from build123d import *

# Parameters (mm, degrees)
SKETCH1_W           = 1090
SKETCH1_H           = 20
BOSS_EXTRUDE1_DEPTH = 1
BOSS_EXTRUDE4_DEPTH = 1090
SKETCH5_W           = 1090
SKETCH5_H           = 1
BOSS_EXTRUDE5_DEPTH = 582
BOSS_EXTRUDE6_DEPTH = 1090
SKETCH7_W           = 1089
SKETCH7_H           = 1
BOSS_EXTRUDE7_DEPTH = 106


with BuildPart() as part:
    # Sketch1 → Boss-Extrude1 (new body)
    with BuildSketch(Plane(origin=(0, 0, 0), x_dir=(1, 0, 0), z_dir=(0, 1, 0))):
        Rectangle(SKETCH1_W, SKETCH1_H)
    extrude(amount=BOSS_EXTRUDE1_DEPTH)

    # Sketch4 → Boss-Extrude4 (add)
    with BuildSketch(Plane.ZY.offset(545)):
        with BuildLine():
            Line((-10, 1), (-10.77384021, 0.366619127))
            ThreePointArc((-10.77384021, 0.366619127), (-10.428146661, 0.096290735), (-10, 0))
            Line((-10, 0), (-10, 1))
        make_face()
    extrude(amount=-BOSS_EXTRUDE4_DEPTH)

    # Sketch5 → Boss-Extrude5 (add)
    with BuildSketch(Plane(origin=(0, 5.500184543, -4.501848885), x_dir=(1, 0, 0), z_dir=(0, 0.7738402097265024, -0.6333808726275547))):
        with Locations((0, 7.605021225)):
            Rectangle(SKETCH5_W, SKETCH5_H)
    extrude(amount=BOSS_EXTRUDE5_DEPTH)

    # Sketch6 → Boss-Extrude6 (add)
    with BuildSketch(Plane(origin=(545, 0, 0), x_dir=(0, 0, -1), z_dir=(1, 0, 0))):
        with BuildLine():
            Line((378.627667869, 451.375002061), (379.627667869, 451.375002061))
            ThreePointArc((379.627667869, 451.375002061), (379.569432227, 451.038728519), (379.401508079, 450.741621188))
            Line((379.401508079, 450.741621188), (378.627667869, 451.375002061))
        make_face()
    extrude(amount=-BOSS_EXTRUDE6_DEPTH)

    # Sketch7 → Boss-Extrude7 (add)
    with BuildSketch(Plane(origin=(0, 451.375002061, 0), x_dir=(1, 0, 0), z_dir=(0, 1, 0))):
        with Locations((0.5, 379.127667869)):
            Rectangle(SKETCH7_W, SKETCH7_H)
    extrude(amount=BOSS_EXTRUDE7_DEPTH)


solid = part.part
Input: part model. Units: mm. Frame: model coordinates. A direction names the side the tool comes from. Round coordinates to 2 decimals unless told otherwise and drop trailing zeros. Loops run counter-clockwise (first coordinate to the right, second up) from the corner with the lowest first, then second, coordinate; pieces in that order, holes last. Notation, with made-up numbers: (28, 72.25) -> (77, 72.25) arc R30 ccw to (77, 98.25) -> close; hole circle Ø8 at (3.25, 26.25). An arc over 180 degrees is marked (long way). Answer as a JSON object with one key per item and string values. Group by question number.
1) Pin query (flat end, axial travel): pin 1 (12 mm diameter, centred on x = -92, z = -243, fed in from +Y); pin 2 (0.5 mm diameter, centred on x = -544.5, z = -379, fed in from +Y) (3 decimals); pin 3 (12 mm diameter, centred on x = 100.5, z = -102, fed in from -Y). Return the tip coordinate at first contact, or that it passes through.
2) Reachability of faces 1 (the flat face through (-8, 0, 0)), 2 (the flat face through (-8, 1, 0)) from +Z, -Z, +X, -X, +Y, -Y: full face, straight path, thin tool, end or side. Return the list, or none.
3) Ray query, L1, parallel to Z at x = 193, y = 515.5; L2, parallel to Y at x = 340.5, z = -83; L3, parallel to Y at x = 304, z = -221. Return the intervals inside material, ascending.
4) Section query A-A on x = -269.5. Output: boundary loops of the cut face in (y, z) (1 decimal).
5) Section query C-C on z = -115.5. Output: boundary loops of the cut face in (x, y), plus the area to 3 significant figures.
6) Section query B-B on y = 258.5. Output: boundary loops of the cut face in (x, z), plus the area to 3 significant figures.
Reply:
{
 "1": {"pin 1": "stops at y = 293", "pin 2": "stops at y = 451.375", "pin 3": "stops at y = 104.49"},
 "2": {"face 1": "+Z, -Z, +X, -X, -Y", "face 2": "+Z, +X, -X, +Y"},
 "3": {"L1": "z = -379.63 to -378.63", "L2": "y = 88.61 to 90.19", "L3": "y = 257.21 to 258.79"},
 "4": {"outline": "(0, -10) arc R1 ccw to (0.4, -10.8) -> (450.7, -379.4) arc R1 ccw to (451.4, -379.6) -> (557.4, -379.6) -> (557.4, -378.6) -> (451.4, -378.6) -> (1, -10) -> (1, 10) -> (0, 10) -> close"},
 "5": {"outline": "(-545, 128.32) -> (545, 128.32) -> (545, 129.9) -> (-545, 129.9) -> close", "area": "1,720 mm2"},
 "6": {"outline": "(-545, -222.05) -> (545, -222.05) -> (545, -220.76) -> (-545, -220.76) -> close", "area": "1,410 mm2"}
}
